from build123d import *

# Parameters (mm, degrees)
SKETCH4_W          = 0.635
SKETCH4_H          = 6.35
CUT_EXTRUDE2_DEPTH = 6.35
CIRPATTERN1_COUNT  = 30


with BuildPart() as part:
    # Sketch3 → Revolve1 (revolve)
    with BuildSketch(Plane.XY, mode=Mode.PRIVATE) as revolve1_sk:
        Polygon((-38.1, 16.300354852), (-38.1, 11.220354852), (-19.05, 11.220354852), (-19.05, 1.695354852), (-15.24, 1.695354852), (-15.24, -1.479645148), (-19.05, -1.479645148), (-19.05, -10.465654768), (-12.065, -14.179645148), (-12.065, -56.089645148), (0, -56.089645148), (0, -52.279645148), (-9.525, -52.279645148), (-9.525, 16.300354852), align=None)
    revolve(revolve1_sk.sketch.rotate(Axis((0, 0, 0), (0, 1, 0)), 270), axis=Axis((0, 0, 0), (0, 1, 0)))

    # Sketch4 → Cut-Extrude2 (cut)
    with BuildSketch(Plane(origin=(12.065, 0, 0), x_dir=(0, 0, -1), z_dir=(1, 0, 0))):
        with Locations((0, -47.199645148)):
            Rectangle(SKETCH4_W, SKETCH4_H)
    cut_extrude2 = extrude(amount=-CUT_EXTRUDE2_DEPTH, mode=Mode.SUBTRACT)

    # CirPattern1: Cut-Extrude2 ×30 about axis
    cirpattern1_axis = Axis((0, 0, 0), (0, 1, 0))
    for i in range(1, CIRPATTERN1_COUNT):
        add(cut_extrude2.rotate(cirpattern1_axis, i * 360 / CIRPATTERN1_COUNT), mode=Mode.SUBTRACT)


solid = part.part
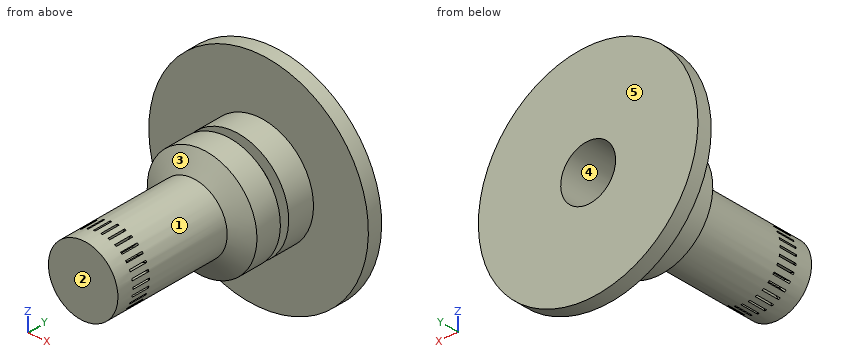
Could you check a few things on this model? Use its own coordinates, in mm. Face numbers are marked on the shaded views. A direction names the side the tool comes from. Round coordinates to 2 decimals unless told otherwise and drop trailing zeros. Order: outer loops, then holes, each group sorted by start corner. A loop starts at its lowest first (then second) coordinate and runs counter-clockwise, first axis right, second up.
Q1. Imagine slicing it at A-A, the plane y = 5. List the corners of the cut face in (x, z) for me (3 decimals), then the cut area to 3 significant figures.
Geometry says:
outline: circle Ø38.1 at (0, 0); hole circle Ø19.05 at (0, 0)
area: 855 mm2
Q2. Imagine slicing it at C-C, the plane x = 29. List the corners of the cut face in (y, z) for me.
Geometry says:
outline: (11.22, -24.71) - (16.3, -24.71) - (16.3, 24.71) - (11.22, 24.71) - close
Q3. Which directions (+Z, -Z, +X, -X, +Y, -Y) give clear straight access to the entire face, cutting with the end or side of a thin tool? Please do the marked faces 1 and 2.
Geometry says:
face 1: -Y
face 2: +Z, -Z, +X, -X, -Y
Q4. Imagine slicing it at B-B, the plane y = -49. State how many separate pieces and enclosed holes the cut face has, then the cut area to 3 significant figures.
Geometry says:
separate pieces: 30
enclosed holes: 0
area: 124 mm2
Q5. Please list where these lines run through material, in increasing order: probe 1 along X at (y, z) = (-23, 0) (3 decimals); probe 2 along Y at (x, z) = (-10, 19.5); probe 3 along Z at (x, y) = (8.5, -32.5).
Geometry says:
probe 1: x = -12.065 to -9.525, 9.525 to 12.065
probe 2: y = 11.22 to 16.3
probe 3: z = -8.56 to -4.3, 4.3 to 8.56
Q6. I'm going to push flat-ended pins straight in: P1, Ø5, axis at x = -18.5, y = -14.5, coming from the -Z side; P2, Ø2, axis at x = 7.5, y = -4, coming from the +Z side; P3, Ø6, axis at x = 4.5, z = 17, coming from the -Y side; P4, Ø12, axis at x = 8.5, y = -2.5, coming from the +Z side. Where does each tip first touch, or does it pass through?
Geometry says:
P1: passes through
P2: stops at z = 17.91
P3: stops at y = -12.84
P4: stops at z = 18.89
Q7. Imagine slicing it at D-D, the plane y = -22. List the corners of the cut face in (x, z) for me (3 decimals).
Geometry says:
outline: circle Ø24.13 at (0, 0); hole circle Ø19.05 at (0, 0)
Q8. Thinking about a two-plate mould opening in X: for the marked faces 3, 4 and 5, which applies, released by +X, released by -X, zero draft, split by the parting line, or undercut?
Geometry says:
face 3: split by the parting line
face 4: undercut
face 5: zero draft
